Check sheet for the drawn part. Datum: minimum x, y, z corner. Units: mm. A direction names the side the tool comes from. Coordinates: 2 decimals unless noted, no trailing zeros. Loops run counter-clockwise (first coordinate to the right, second up) from the corner with the lowest first, then second, coordinate; pieces in that order, holes last. Notation, with made-up numbers: (89, 86) - (122, 86) arc R5 ccw to (122, 95) - close; hole circle Ø10 at (-5, 47). An arc over 180 degrees is marked (long way). Answer as CSV lines item,"result". Start each with the question number.
1. Cross-section at C-C (y = 2.05). Enter the section's corners in (x, z).
2. Gauge pin test, flat ends, axial feed: P1, Ø1.8, axis at x = 17.5, z = 2.5, coming from the -Y side; P2, Ø1.5, axis at x = 2.5, y = 1, coming from the -Z side. Record the tip position at first contact, or that the pin passes through.
3. Material ranges on line 1 (Z direction, x = 17.5, y = 2.95); line 2 (X direction, y = 2.7, z = 1.4); line 3 (Y direction, x = 12, z = 1.4), recorded low to high. Write a range as [from, to].
4. Cross-section at A-A (x = 2.5). Enter the section's corners in (y, z).
5. Cross-section at B-B (z = 4.25). Enter the section's corners in (x, y), plus the area to 3 significant figures.
6. Release check for a two-part mould opening along Z. For the marked faces 1, 2 and 3 record: pulls with the +Z half, pulls with the -Z half, needs draft (parallel to the pull), parting line crosses it, or undercut.
7. Set-up check for the marked faces 4 and 5: record each of +Z, -Z, +X, -X, +Y, -Y from which the full face is reachable in a straight line by a thin tool's end or side.
8. Cross-section at D-D (z = 3.35). Enter the section's corners in (x, y).
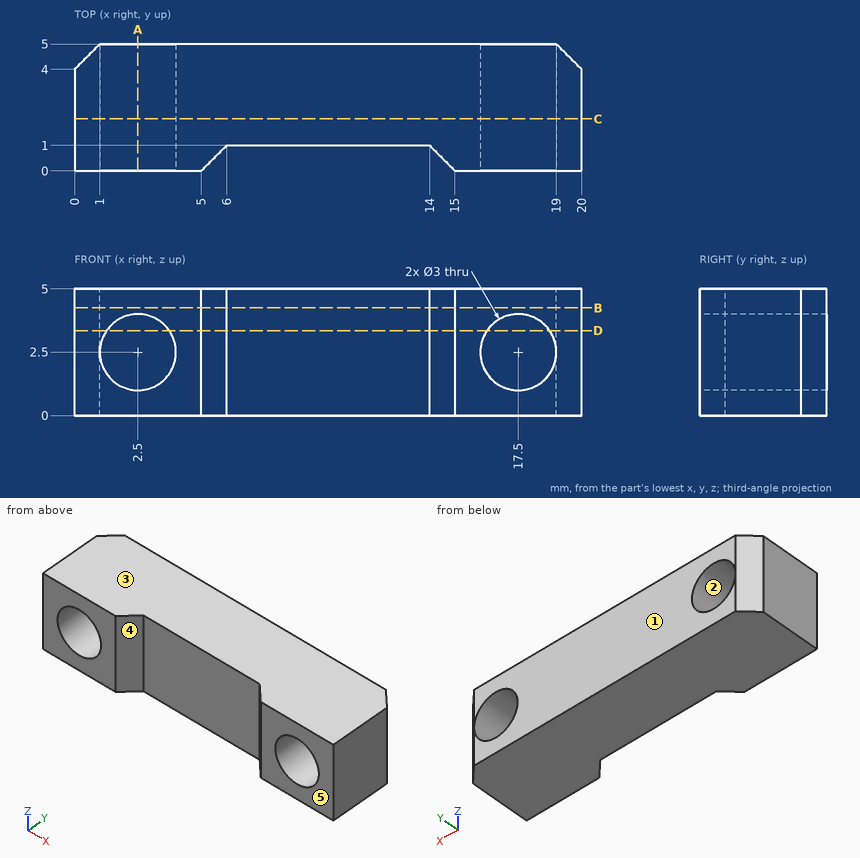
Values follow:
1,outline,"(0, 0) - (20, 0) - (20, 5) - (0, 5) - close; hole circle Ø3 at (2.5, 2.5); hole circle Ø3 at (17.5, 2.5)"
2,P1,"passes through"
2,P2,"stops at z = 0"
3,line 1,"z = [0, 1], [4, 5]"
3,line 2,"x = [0, 1.48], [3.52, 16.48], [18.52, 20]"
3,line 3,"y = [1, 5]"
4,outline,"(0, 0) - (5, 0) - (5, 1) - (0, 1) - close; (0, 4) - (5, 4) - (5, 5) - (0, 5) - close"
5,outline,"(0, 0) - (5, 0) - (6, 1) - (14, 1) - (15, 0) - (20, 0) - (20, 4) - (19, 5) - (1, 5) - (0, 4) - close"
5,area,"90.0 mm²"
6,face 1,"needs draft"
6,face 2,"undercut"
6,face 3,"pulls with the +Z half"
7,face 4,"+Z, -Z, -Y"
7,face 5,"+Z, -Z, +X, -X, -Y"
8,outline,"(0, 0) - (1.26, 0) - (1.26, 5) - (1, 5) - (0, 4) - close; (3.74, 0) - (5, 0) - (6, 1) - (14, 1) - (15, 0) - (16.26, 0) - (16.26, 5) - (3.74, 5) - close; (18.74, 0) - (20, 0) - (20, 4) - (19, 5) - (18.74, 5) - close"
